Design review of the part built by this model. Coordinates are the model's own, in mm. A direction names the side the tool comes from. Round coordinates to 2 decimals unless told otherwise and drop trailing zeros. Write each loop counter-clockwise with the first axis right and the second up, starting at its lowest first coordinate (ties: lowest second). Pieces come first, ordered by that corner, then holes. Notation, with made-up numbers: M 38.25,2 L 82.25,2 A26 ccw 82.25,40 Z; hole C 83,12.5 d4. An arc over 180 degrees is marked long. Use CSV: the item, a comma, the result in double quotes.
from build123d import *

# Parameters (mm, degrees)
F0_W     = 380
F0_H     = 380
F1_DEPTH = 350
F2_W     = 342
F2_H     = 312
F3_DEPTH = 361
F4_R     = 20
F5_DEPTH = 25


with BuildPart() as f1:
    # F0 (on Top) → F1 (new body)
    with BuildSketch(Plane.XY):
        Rectangle(F0_W, F0_H)
    extrude(amount=F1_DEPTH)

    # F2 (on face) → F3 (cut)
    with BuildSketch(Plane.XZ.offset(190)):
        with Locations((0, 175)):
            Rectangle(F2_W, F2_H)
    extrude(amount=-F3_DEPTH, mode=Mode.SUBTRACT)

    # F4 (on face) → F5 (join)
    with BuildSketch(Plane.XY):
        with Locations((169.437533, -169.759312)):
            Circle(F4_R)
        with Locations((169.437532, 170.240688)):
            Circle(F4_R)
        with Locations((-170.562468, 170.240687)):
            Circle(F4_R)
        with Locations((-170.562467, -169.759313)):
            Circle(F4_R)
    extrude(amount=-F5_DEPTH)


solid = f1.part
1) Machinability: for faces 1 (the face through (-3, 3, 350)), 2 (the face through (-3, 3, 0)), 3 (the face through (-186, 186, 0)), 4 (the face through (171, -12, 173)), which of the approach directions +Z, -Z, +X, -X, +Y, -Y give a long, thin tool a straight path to every point of the face, cutting with its end or side? Answer none if there is none.
Answers:
face 1,"+Z, +X, -X, +Y, -Y"
face 2,"-Z"
face 3,"-Z, -X, +Y"
face 4,"-Y"
2) Add section A-A on y = 22. Write out the cut boundary in (x, z).
Answers:
outline,"M -190,0 L 190,0 L 190,350 L -190,350 Z; hole M -171,19 L 171,19 L 171,331 L -171,331 Z"
3) For pin 1 Ø1 at (y, z) = (-53.5, 285.5) entering from -X; pin 2 Ø3 at (x, y) = (-152, 92) entering from -Z; pin 3 Ø4 at (x, z) = (-20, 267.5) entering from -Y, all flat-tipped, find the tip position at first contact; note any pin that passes through.
Answers:
pin 1,"x = -190"
pin 2,"z = 0"
pin 3,"y = 171"
4) Add section B-B on z = 221. Write out the cut boundary in (x, y), then the cut area to 3 significant figures.
Answers:
outline,"M -190,-190 L -171,-190 L -171,171 L 171,171 L 171,-190 L 190,-190 L 190,190 L -190,190 Z"
area,"20,900 mm²"
5) Add section C-C on x = 125.5. Write out the cut boundary in (y, z).
Answers:
outline,"M -190,0 L 190,0 L 190,350 L -190,350 L -190,331 L 171,331 L 171,19 L -190,19 Z"
6) Wall thickness on line 1 along Z through (x, y) = (-162, -5); line 2 along X through (y, z) = (-141.5, 111.5); line 3 along Y through (x, z) = (43, 307): over which ranges is each line inside the solid? List them lowest first. Write a range as [from, to].
Answers:
line 1,"[0, 19], [331, 350]"
line 2,"[-190, -171], [171, 190]"
line 3,"[171, 190]"
7) The part is to be moulded in two halves that separate along X. For faces 5 (the face through (-171, -169, -25)), 6 (the face through (166.83, -149.93, -12.32)), 7 (the face through (-190, -3, 173)), 8 (the face through (190, -3, 173)), say which applies: released by +X, released by -X, zero draft, split by the parting line, or undercut.
Answers:
face 5,"zero draft"
face 6,"undercut"
face 7,"released by -X"
face 8,"released by +X"
